Check sheet for the drawn part. Datum: minimum x, y, z corner. Units: mm. A direction names the side the tool comes from. Give positions to 0.01 mm unless a question says otherwise; leave off trailing zeros. Order: outer loops, then holes, each group sorted by start corner. A loop starts at its lowest first (then second) coordinate and runs counter-clockwise, first axis right, second up. Notation, with made-up numbers: (25, 45.25) - (83, 45.25) arc R20 cw to (83, 55.25) - close; hole circle Ø1 at (28.25, 41). An arc over 180 degrees is marked (long way). Answer as a JSON object with one key per item and string values. Group by question number.
(1) Thickness scan on line 1 (Z direction, x = 66.5, y = 7.25); line 2 (Z direction, x = 5, y = 6.5); line 3 (Y direction, x = 3.5, z = 12.7). Record the ranges inside material, lowest first.
(2) Access from +Z, -Z, +X, -X, +Y, -Y to the whole of each face (thin tool, end or side, straight path). Record for the marked faces 4, 5, 6, 7 and 8.
(3) Section check A-A (x = 64). Record the boundary of the cut face in (y, z), then the cut area to 3 significant figures.
(4) Depth check by flat-ended pin: pin 1 Ø3 at (x, y) = (26.5, 6.5) entering from +Z; pin 2 Ø3 at (y, z) = (5.5, 12) entering from +X; pin 3 Ø1.5 at (y, z) = (5, 5.5) entering from -X; pin 4 Ø1.8 at (x, y) = (3.5, 5) entering from -Z. Enter the tip coordinate at first touch or a pass-through.
(5) Section check D-D (x = 3.5). Record the boundary of the cut face in (y, z).
(6) Mould release check, pull along X, two halves, no side actions. Record for the marked faces 1, 2 and 3: +X half, -X half, draft (parallel to the pull), parting line (faces both ways), or undercut.
(7) Section check C-C (y = 5). Count the separate pieces of the cut face and the enclosed holes in it, then the cut area to 3 significant figures.
(8) Section check B-B (z = 16.75). Record the boundary of the cut face in (x, y), then the cut area to 3 significant figures.
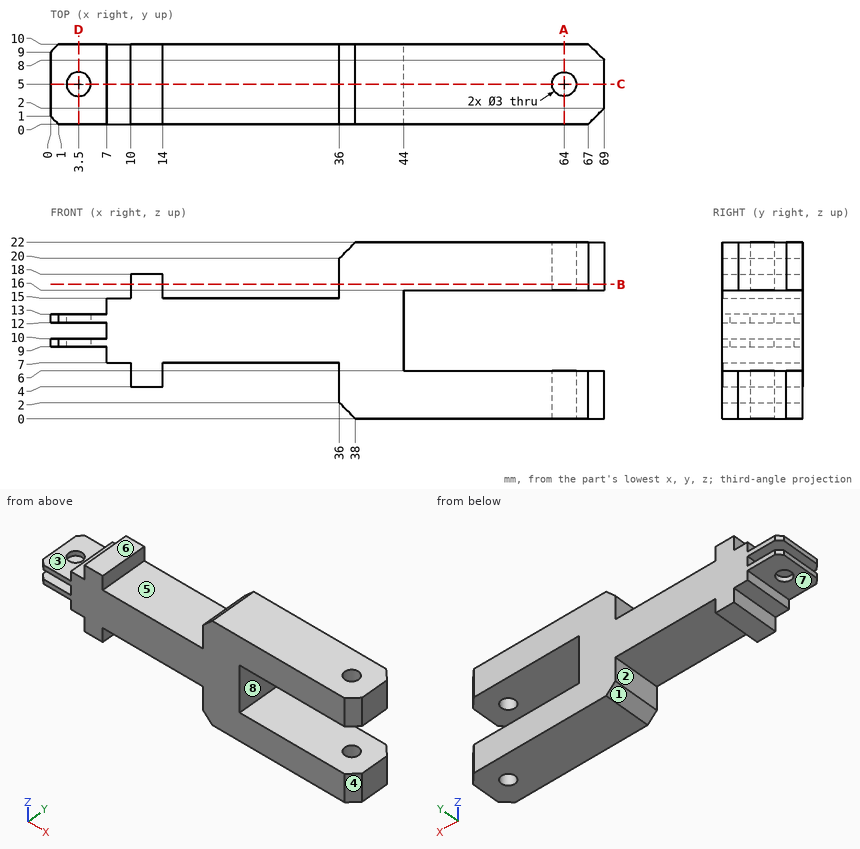
Solutions:
{
 "1": {"line 1": "z = 0 to 6, 16 to 22", "line 2": "z = 9 to 10, 12 to 13", "line 3": "y = 0 to 3.5, 6.5 to 10"},
 "2": {"face 4": "+Z, -Z, +X, -Y", "face 5": "+Z, +Y, -Y", "face 6": "+Z, -X, +Y, -Y", "face 7": "-Z, -X, +Y, -Y", "face 8": "+X, +Y, -Y"},
 "3": {"outline": "(0, 0) - (3.5, 0) - (3.5, 6) - (0, 6) - close; (0, 16) - (3.5, 16) - (3.5, 22) - (0, 22) - close; (6.5, 0) - (10, 0) - (10, 6) - (6.5, 6) - close; (6.5, 16) - (10, 16) - (10, 22) - (6.5, 22) - close", "area": "84.0 mm2"},
 "4": {"pin 1": "stops at z = 15", "pin 2": "stops at x = 44", "pin 3": "stops at x = 10", "pin 4": "passes through"},
 "5": {"outline": "(0, 9) - (3.5, 9) - (3.5, 10) - (0, 10) - close; (0, 12) - (3.5, 12) - (3.5, 13) - (0, 13) - close; (6.5, 9) - (10, 9) - (10, 10) - (6.5, 10) - close; (6.5, 12) - (10, 12) - (10, 13) - (6.5, 13) - close"},
 "6": {"face 1": "-X half", "face 2": "undercut", "face 3": "draft"},
 "7": {"separate pieces": "5", "enclosed holes": "0", "area": "700 mm2"},
 "8": {"outline": "(10, 0) - (14, 0) - (14, 10) - (10, 10) - close; (36, 0) - (67, 0) - (69, 2) - (69, 8) - (67, 10) - (36, 10) - close; hole circle Ø3 at (64, 5)", "area": "359 mm2"}
}
